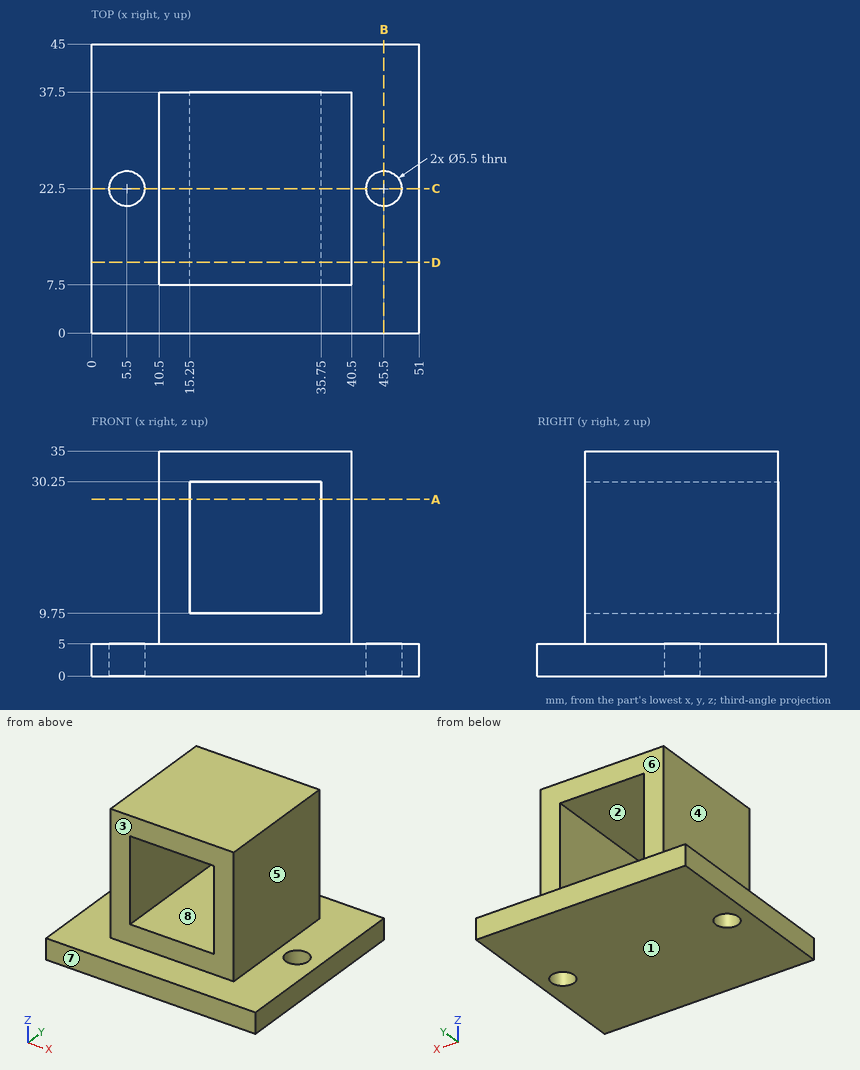
Study the drawing (mm; zero at the part's minimum x, y, z) and answer. A direction names the side the tool comes from. Round coordinates to 2 decimals unless told otherwise and drop trailing zeros. Loops run counter-clockwise (first coordinate to the right, second up) from the corner with the lowest first, then second, coordinate; pieces in that order, holes last. Notation, with made-up numbers: (-31.75, 53) -> (-19.75, 53) arc R21 ccw to (-19.75, 73) -> close; hole circle Ø9 at (15.5, -38.5). An arc over 180 degrees is marked (long way). One line per item, written item: value.
1) A cutting plane is placed at D-D (y = 11). Determine the outline of the cut face in (x, z), and give its area (3 significant figures).
Answer list:
outline: (0, 0) -> (51, 0) -> (51, 5) -> (40.5, 5) -> (40.5, 35) -> (10.5, 35) -> (10.5, 5) -> (0, 5) -> close; hole (15.25, 9.75) -> (35.75, 9.75) -> (35.75, 30.25) -> (15.25, 30.25) -> close
area: 735 mm²
2) For the marked faces 4, 5, 6, 7 and 8, determine the directions among +Z, -Z, +X, -X, +Y, -Y from which every point of the face is accessible in a straight line to the end or side of a thin tool.
Answer list:
face 4: +Z, -X, +Y, -Y
face 5: +Z, +X, +Y, -Y
face 6: +Z, +X, -X, +Y
face 7: +Z, -Z, +X, -X, -Y
face 8: +Y, -Y
3) A cutting plane is placed at C-C (y = 22.5). Determine the outline of the cut face in (x, z), and give its area (3 significant figures).
Answer list:
outline: (0, 0) -> (2.75, 0) -> (2.75, 5) -> (0, 5) -> close; (8.25, 0) -> (42.75, 0) -> (42.75, 5) -> (40.5, 5) -> (40.5, 35) -> (10.5, 35) -> (10.5, 5) -> (8.25, 5) -> close; (48.25, 0) -> (51, 0) -> (51, 5) -> (48.25, 5) -> close; hole (15.25, 9.75) -> (35.75, 9.75) -> (35.75, 30.25) -> (15.25, 30.25) -> close
area: 680 mm²
4) Consider L1, parallel to X at y = 9, z = 18; L2, parallel to Y at x = 5.5, z = 3.1; L3, parallel to X at y = 22, z = 2. Determine where each line is inside the solid, lowest interval first. Write a range as [from, to].
Answer list:
L1: x = [10.5, 15.25], [35.75, 40.5]
L2: y = [0, 19.75], [25.25, 45]
L3: x = [0, 2.8], [8.2, 42.8], [48.2, 51]
5) The mould has two halves that part along Z. Classify the marked faces 1, 2 and 3: pulls with the +Z half, pulls with the -Z half, needs draft (parallel to the pull), parting line crosses it, or undercut.
Answer list:
face 1: pulls with the -Z half
face 2: undercut
face 3: needs draft
6) Flat-ended cylindrical pins translate along their axes: P1, Ø6.5, axis at x = 45.5, y = 22.5, coming from the +Z side; P2, Ø3, axis at x = 12.5, z = 22.5, coming from the -Y side; P3, Ø12, axis at x = 7, z = 21.5, coming from the +Y side; P4, Ø15, axis at x = 23.5, z = 21.5, coming from the +Y side. Find the tip coordinate at first contact, or state that the pin passes through.
Answer list:
P1: stops at z = 5
P2: stops at y = 7.5
P3: stops at y = 37.5
P4: passes through
7) A cutting plane is placed at A-A (z = 27.5). Determine the outline of the cut face in (x, y).
Answer list:
outline: (10.5, 7.5) -> (15.25, 7.5) -> (15.25, 37.5) -> (10.5, 37.5) -> close; (35.75, 7.5) -> (40.5, 7.5) -> (40.5, 37.5) -> (35.75, 37.5) -> close
8) A cutting plane is placed at B-B (x = 45.5). Determine the outline of the cut face in (y, z).
Answer list:
outline: (0, 0) -> (19.75, 0) -> (19.75, 5) -> (0, 5) -> close; (25.25, 0) -> (45, 0) -> (45, 5) -> (25.25, 5) -> close
